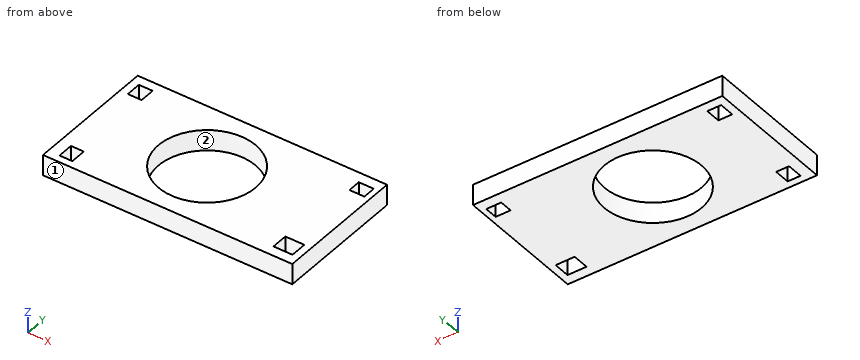
from build123d import *

# Parameters (mm, degrees)
F0_W      = 306.200504303
F0_H      = 160.9693467617
F1_DEPTH  = 25.4
F2_W      = 16.9635862112
F2_H      = 18.7774226069
F2_W_2    = 18.3757990599
F2_H_2    = 15.9212723374
F2_W_3    = 15.8156380057
F2_H_3    = 19.4401964545
F3_DEPTH  = 25.4
F4_W      = 23.3820155263
F4_H      = 20.1737955213
F5_DEPTH  = 25.4
F10_W     = 156.8522006273
F10_H     = 128.1716823578
F10_W_2   = 155.7295322418
F10_H_2   = 9.3674659729
F11_DEPTH = 25.4
F12_R     = 59.7527814568
F13_DEPTH = 25.4


# Not quite as in the source:
# - a feature of the source that left no trace in its solid (it failed there, or was rolled back) is left out


with BuildPart() as f1:
    # F0 (on Top) → F1 (new body)
    with BuildSketch(Plane.XY):
        Rectangle(F0_W, F0_H)
    extrude(amount=F1_DEPTH)

    # F2 (on face) → F3 (cut)
    with BuildSketch(Plane.XY.offset(25.4)):
        with Locations((-134.9064931273, 59.5765523612)):
            Rectangle(F2_W, F2_H)
        with Locations((137.0917782187, 59.4723559916)):
            Rectangle(F2_W_2, F2_H_2)
        with Locations((-131.3789226115, -61.8558935821)):
            Rectangle(F2_W_3, F2_H_3)
    extrude(amount=-F3_DEPTH, mode=Mode.SUBTRACT)

    # F4 (on face) → F5 (cut)
    with BuildSketch(Plane.XY.offset(25.4)):
        with Locations((132.6544694602, -57.8851737082)):
            Rectangle(F4_W, F4_H)
    extrude(amount=-F5_DEPTH, mode=Mode.SUBTRACT)

    # F10 (on Right) → F11 (cut)
    with BuildSketch(Plane.YZ):
        with Locations((274.1180285811, -160.389393568)):
            Rectangle(F10_W, F10_H)
        with Locations((-275.496006012, 285.2313816547)):
            Rectangle(F10_W_2, F10_H_2)
    extrude(amount=-F11_DEPTH, mode=Mode.SUBTRACT)

    # F12 (on face) → F13 (cut)
    with BuildSketch(Plane.XY.offset(25.4)):
        with Locations((-9.737694636, 0)):
            Circle(F12_R)
    extrude(amount=-F13_DEPTH, mode=Mode.SUBTRACT)


solid = f1.part
Source: CAD feature listing. Evaluate the final solid. Frame: model axes, mm. Face numbers are marked on the shaded views. Give positions to 0.01 mm unless a question says otherwise; leave off trailing zeros. Write each loop counter-clockwise with the first axis right and the second up, starting at its lowest first coordinate (ties: lowest second). Pieces come first, ordered by that corner, then holes. Notation, with made-up numbers: M 48.25,88 L 55.25,88 A29 cw 55.25,116 Z; hole C 65,-35 d8. An arc over 180 degrees is marked long. Answer as a JSON object with one key per item and string values.
Q1. Cut plane B-B, the plane y = 0. Return the cut outline in (x, z), then the cut area to 3 significant figures.
Geometry check:
{"outline": "M -153.1,0 L -69.49,0 L -69.49,25.4 L -153.1,25.4 Z; M 50.02,0 L 153.1,0 L 153.1,25.4 L 50.02,25.4 Z", "area": "4,740 mm^2"}
Q2. Ray query, line 1 along Y through (x, z) = (129, 22.25); line 2 along Y through (x, z) = (-133.5, 17.25); line 3 along X through (y, z) = (52, 1.5). Return the intervals inside material, ascending.
Geometry check:
{"line 1": "y = -80.48 to -67.97, -47.8 to 51.51, 67.43 to 80.48", "line 2": "y = -80.48 to -71.58, -52.14 to 50.19, 68.97 to 80.48", "line 3": "x = -153.1 to -143.39, -126.42 to -39.17, 19.7 to 127.9, 146.28 to 153.1"}
Q3. Cut plane D-D, the plane z = 13.25. Return the cut outline in (x, y), then the cut area to 3 significant figures.
Geometry check:
{"outline": "M -153.1,-80.48 L 153.1,-80.48 L 153.1,80.48 L -153.1,80.48 Z; hole M -143.39,50.19 L -126.42,50.19 L -126.42,68.97 L -143.39,68.97 Z; hole M -139.29,-71.58 L -123.47,-71.58 L -123.47,-52.14 L -139.29,-52.14 Z; hole C -9.74,0 d119.51; hole M 120.96,-67.97 L 144.35,-67.97 L 144.35,-47.8 L 120.96,-47.8 Z; hole M 127.9,51.51 L 146.28,51.51 L 146.28,67.43 L 127.9,67.43 Z", "area": "36,700 mm^2"}
Q4. Contact query for a flat-ended pin moving along its axis: P1, Ø5, axis at x = 41, y = -36, coming from the -Z side. Output: stop coordinate, or through.
Geometry check:
{"P1": "stops at z = 0"}
Q5. Cut plane A-A, the plane y = -65. Return the cut outline in (x, z).
Geometry check:
{"outline": "M -153.1,0 L -139.29,0 L -139.29,25.4 L -153.1,25.4 Z; M -123.47,0 L 120.96,0 L 120.96,25.4 L -123.47,25.4 Z; M 144.35,0 L 153.1,0 L 153.1,25.4 L 144.35,25.4 Z"}
Q6. Cut plane C-C, the plane x = 30.5. Return the cut outline in (y, z), then the cut area to 3 significant figures.
Geometry check:
{"outline": "M -80.48,0 L -44.17,0 L -44.17,25.4 L -80.48,25.4 Z; M 44.17,0 L 80.48,0 L 80.48,25.4 L 44.17,25.4 Z", "area": "1,840 mm^2"}
Q7. Mould query, pull axis X, two halves, no side actions, for the marked faces 1 and 2. Classes: +X half, -X half, draft (parallel to the pull), parting line (faces both ways), or undercut.
Geometry check:
{"face 1": "draft", "face 2": "undercut"}
